```python
from build123d import *

# Parameters (mm, degrees)
F0_W     = 24
F0_H     = 21
F1_DEPTH = 5
F2_R     = 2


# Not quite as in the source:
# - a feature of the source that left no trace in its solid (it failed there, or was rolled back) is left out


with BuildPart() as f1:
    # F0 (on Front) → F1 (new body)
    with BuildSketch(Plane.XZ):
        with Locations((-12, 10.5)):
            Rectangle(F0_W, F0_H)
    extrude(amount=F1_DEPTH)

    # F2
    f2_edges = [f1.edges().sort_by_distance(p)[0] for p in [
        (-12, -5, 0),
        (0, -5, 10.5),
        (-12, -5, 21),
        (-24, -5, 10.5),
    ]]
    fillet(f2_edges, radius=F2_R)


solid = f1.part
```
Can you work these out from the model? Positions are in its coordinate system, mm. Coordinates: 2 decimals unless noted, no trailing zeros. Order: outer loops, then holes, each group sorted by start corner. A loop starts at its lowest first (then second) coordinate and runs counter-clockwise, first axis right, second up.
1. I need wall thicknesses on line 1 (X direction, y = -4.7, z = 11.5); line 2 (Y direction, x = -2.5, z = 1.5); line 3 (X direction, y = -3.8, z = 8). Which ranges of each line are inside material? Lowest first, please.
2. If we section it at B-B (y = -3.7): Please give me the cut outline in (x, z), then the cut area to 3 significant figures.
3. If we section it at A-A (x = -3.75): Please give me the cut outline in (y, z).
Entries:
1. line 1: x = -23.05 to -0.95
1. line 2: y = -4.94 to 0
1. line 3: x = -23.83 to -0.17
2. outline: (-23.87, 0.13) - (-0.13, 0.13) - (-0.13, 20.87) - (-23.87, 20.87) - close
2. area: 493 mm2
3. outline: (-5, 2) arc R2 ccw to (-3, 0) - (0, 0) - (0, 21) - (-3, 21) arc R2 ccw to (-5, 19) - close
